```python
from build123d import *

# Parameters (mm, degrees)
SKETCH1_W           = 12
SKETCH1_H           = 4.6
BOSS_EXTRUDE1_DEPTH = 12
SKETCH2_W           = 15.2
SKETCH2_H           = 7.25
BOSS_EXTRUDE2_DEPTH = 21
FILLET1_R           = 3.5
BOSS_EXTRUDE3_START = -0.952452
SKETCH4_W           = 5
SKETCH4_H           = 5
BOSS_EXTRUDE3_DEPTH = 7.452452
FILLET2_R           = 0.5
FILLET3_R           = 0.5


with BuildPart() as part:
    # Sketch1 → Boss-Extrude1 (new body)
    with BuildSketch(Plane.XY):
        with Locations((6, 2.3)):
            Rectangle(SKETCH1_W, SKETCH1_H)
    extrude(amount=BOSS_EXTRUDE1_DEPTH)

    # Sketch2 → Boss-Extrude2 (add)
    with BuildSketch(Plane(origin=(0, 0, 0), x_dir=(-1, 0, 0), z_dir=(0, 0, -1))):
        with Locations((-6, 2.325)):
            Rectangle(SKETCH2_W, SKETCH2_H)
    extrude(amount=BOSS_EXTRUDE2_DEPTH)

    # Fillet1
    fillet1_edges = [part.edges().sort_by_distance(p)[0] for p in [
        (6, -1.3, -21),
        (6, 5.95, -21),
    ]]
    fillet(fillet1_edges, radius=FILLET1_R)

    # Sketch4 → Boss-Extrude3 (add)
    with BuildSketch(Plane(origin=(0, 0, -21), x_dir=(-1, 0, 0), z_dir=(0, 0, -1)).offset(BOSS_EXTRUDE3_START)):
        with Locations((-6, 2.35)):
            Rectangle(SKETCH4_W, SKETCH4_H)
    extrude(amount=BOSS_EXTRUDE3_DEPTH)

    # Sketch5 → Revolve1 (revolve)
    with BuildSketch(Plane(origin=(6, 0, 0), x_dir=(0, 0, -1), z_dir=(1, 0, 0)), mode=Mode.PRIVATE) as revolve1_sk:
        with BuildLine():
            Line((26.35, -2.675), (26.35, 84.325))
            ThreePointArc((26.35, 84.325), (23.891258371, 83.316024239), (22.85, 80.870779161))
            Line((22.85, 80.870779161), (21.75, -2.675))
            Line((21.75, -2.675), (26.35, -2.675))
        make_face()
    revolve(revolve1_sk.sketch.rotate(Axis((6, -2.675, -26.35), (0, 1, 0)), 90), axis=Axis((6, -2.675, -26.35), (0, 1, 0)))

    # Sketch6 → Revolve2 (revolve)
    with BuildSketch(Plane(origin=(6, 0, 0), x_dir=(0, 0, -1), z_dir=(1, 0, 0))):
        Polygon((21, 2.325), (21, 7.325), (15, 5.95), (15, 2.325), align=None)
    revolve(axis=Axis((6, 2.325, -15), (0, 0, -1)))

    # Fillet2
    fillet2_edges = [part.edges().sort_by_distance(p)[0] for p in [
        (13.6, 2.325, -21),
        (-1.6, 2.325, -21),
        (-1.6, 5.95, -8.75),
        (-1.6, -1.3, -8.75),
        (-1.6, 4.924873734, -19.974873734),
        (-1.6, -0.274873734, -19.974873734),
        (13.6, -1.3, -8.75),
        (13.6, 5.95, -8.75),
        (13.6, 4.924873734, -19.974873734),
        (13.6, -0.274873734, -19.974873734),
    ]]
    fillet(fillet2_edges, radius=FILLET2_R)

    # Fillet3
    fillet3_edges = [part.edges().sort_by_distance(p)[0] for p in [
        (0, 4.6, 6),
        (12, 4.6, 6),
        (12, 0, 6),
        (0, 0, 6),
    ]]
    fillet(fillet3_edges, radius=FILLET3_R)


solid = part.part
```
Geometry: final body of the model. Coordinates: model frame, mm. A direction names the side the tool comes from. Round coordinates to 2 decimals unless told otherwise and drop trailing zeros. Order: outer loops, then holes, each group sorted by start corner. A loop starts at its lowest first (then second) coordinate and runs counter-clockwise, first axis right, second up. Notation, with made-up numbers: (-40, -17.75) -> (13, -17.75) arc R27 ccw to (13, 0.25) -> close; hole circle Ø6 at (39, 20.5). An arc over 180 degrees is marked (long way). Use CSV: the item, a comma, the result in double quotes. Start each with the question number.
1) Section C-C (y = 57). Return the cut outline in (x, z), and give its area (3 significant figures).
2) Section D-D (y = 32.5). Return the cut outline in (x, z), and give its area (3 significant figures).
3) Material intervals for line 1 along X through (y, z) = (2.5, 2); line 2 along Y through (x, z) = (9.25, -6); line 3 along Y through (x, z) = (4, 2.5), sorted ascending. Write a range as from..to.
4) Section B-B (z = -10). Return the cut outline in (x, y), and give its area (3 significant figures).
5) Set-up query: faces 5 (the face through (0, 2, 6)), 6 (the face through (9, 2, -21)), 7 (the face through (11.127, 5.339, -19.476)), 8 (the face through (6, 4.6, 6)), 9 (the face through (12, 2, 6)). Return all of +Z, -Z, +X, -X, +Y, -Y with unobstructed straight access to the full face (end or side cutting, diameter ignored); none if empty.
6) First-contact query: pin 1 Ø7 at (x, z) = (8.5, -4.5) entering from -Y; pin 2 Ø1.8 at (y, z) = (3, 3.5) entering from -X; pin 3 Ø1 at (x, y) = (2, 23) entering from +Z. Flat tips, straight axial feed; report the tip coordinate or a pass-through.
7) Section A-A (z = 2). Return the cut outline in (x, y).
8) Draft query along Z for faces 1 (the face through (0.803, -0.689, -19.476)), 2 (the face through (6, 5, 0)), 3 (the face through (0.803, 5.339, -19.476)), 4 (the face through (6, 0, 6)). Return one class per face: +Z half, -Z half, draft (parallel to the pull), parting line (faces both ways), or undercut.
Returned:
1,outline,"circle Ø7.63 at (6, -26.35)"
1,area,"45.7 mm²"
2,outline,"circle Ø8.27 at (6, -26.35)"
2,area,"53.8 mm²"
3,line 1,"x = 0..12"
3,line 2,"y = -1.3..5.95"
3,line 3,"y = 0..4.6"
4,outline,"(-1.6, -0.8) arc R0.5 ccw to (-1.1, -1.3) -> (13.1, -1.3) arc R0.5 ccw to (13.6, -0.8) -> (13.6, 5.45) arc R0.5 ccw to (13.1, 5.95) -> (-1.1, 5.95) arc R0.5 ccw to (-1.6, 5.45) -> close"
4,area,"110 mm²"
5,face 5,"+Z, -X, +Y, -Y"
5,face 6,"none"
5,face 7,"+X, +Y"
5,face 8,"+Z, +X, -X, +Y"
5,face 9,"+Z, +X, +Y, -Y"
6,pin 1,"stops at y = -1.3"
6,pin 2,"stops at x = 0"
6,pin 3,"stops at z = -23.92"
7,outline,"(0, 0.5) arc R0.5 ccw to (0.5, 0) -> (11.5, 0) arc R0.5 ccw to (12, 0.5) -> (12, 4.1) arc R0.5 ccw to (11.5, 4.6) -> (0.5, 4.6) arc R0.5 ccw to (0, 4.1) -> close"
8,face 1,"undercut"
8,face 2,"+Z half"
8,face 3,"undercut"
8,face 4,"draft"
